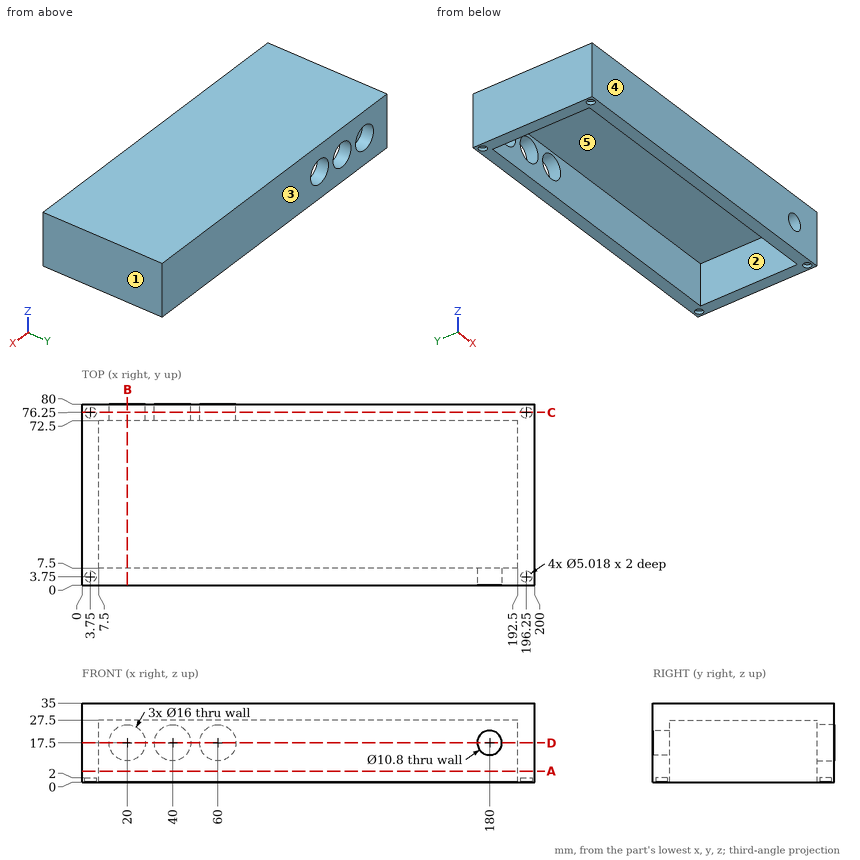
Can you work these out from the drawing? Everything is in mm from the part's minimum corner. A direction names the side the tool comes from. Give positions to 0.01 mm unless a question says otherwise; leave off trailing zeros. Loops run counter-clockwise (first coordinate to the right, second up) from the corner with the lowest first, then second, coordinate; pieces in that order, holes last. Notation, with made-up numbers: (-15, 58.5) -> (-4, 58.5) arc R11 cw to (-4, 70.5) -> close; hole circle Ø1 at (-17.5, 67). An arc over 180 degrees is marked (long way). Put each result on its own line as item: value.
(1) Please list where these lines run through material, in increasing order: probe 1 along X at (y, z) = (75.25, 17.5); probe 2 along X at (y, z) = (76.25, 0.9); probe 3 along X at (y, z) = (29, 16.5). Write a range as [from, to].
Computed:
probe 1: [0, 12], [28, 32], [48, 52], [68, 200]
probe 2: [0, 1.24], [6.26, 193.74], [198.76, 200]
probe 3: [0, 7.5], [192.5, 200]
(2) Imagine slicing it at D-D on z = 17.5. Write out the boundary of the cut face in (x, y).
Computed:
outline: (0, 0) -> (174.6, 0) -> (174.6, 7.5) -> (7.5, 7.5) -> (7.5, 72.5) -> (12, 72.5) -> (12, 80) -> (0, 80) -> close; (28, 72.5) -> (32, 72.5) -> (32, 80) -> (28, 80) -> close; (48, 72.5) -> (52, 72.5) -> (52, 80) -> (48, 80) -> close; (68, 72.5) -> (192.5, 72.5) -> (192.5, 7.5) -> (185.4, 7.5) -> (185.4, 0) -> (200, 0) -> (200, 80) -> (68, 80) -> close
(3) Imagine slicing it at C-C on y = 76.25. Write out the boundary of the cut face in (x, z), plus the area to 3 significant figures.
Computed:
outline: (0, 0) -> (1.24, 0) -> (1.24, 2) -> (6.26, 2) -> (6.26, 0) -> (193.74, 0) -> (193.74, 2) -> (198.76, 2) -> (198.76, 0) -> (200, 0) -> (200, 35) -> (0, 35) -> close; hole circle Ø16 at (20, 17.5); hole circle Ø16 at (40, 17.5); hole circle Ø16 at (60, 17.5)
area: 6,380 mm^2
(4) Imagine slicing it at A-A on z = 5. Write out the boundary of the cut face in (x, y).
Computed:
outline: (0, 0) -> (200, 0) -> (200, 80) -> (0, 80) -> close; hole (7.5, 7.5) -> (192.5, 7.5) -> (192.5, 72.5) -> (7.5, 72.5) -> close
(5) Imagine slicing it at B-B on x = 20. Write out the boundary of the cut face in (y, z).
Computed:
outline: (0, 0) -> (7.5, 0) -> (7.5, 27.5) -> (72.5, 27.5) -> (72.5, 25.5) -> (80, 25.5) -> (80, 35) -> (0, 35) -> close; (72.5, 0) -> (80, 0) -> (80, 9.5) -> (72.5, 9.5) -> close
(6) I'm going to push flat-ended pins straight in: pin 1 Ø12 at (x, z) = (137.5, 31) entering from -Y; pin 2 Ø1.5 at (x, y) = (47.5, 69) entering from -Z; pin 3 Ø1.5 at (x, y) = (195, 76) entering from -Z. Where does each tip first touch, or does it pass through?
Computed:
pin 1: y = 0
pin 2: z = 27.5
pin 3: z = 2
(7) For the marked faces 4 and 5, which set-ups out of +Z, -Z, +X, -X, +Y, -Y let a thin tool reach every point of the face, with its end or its side?
Computed:
face 4: +Z, -Z, +X, -X, -Y
face 5: -Z
(8) Thinking about a two-plate mould opening in Y: for the marked faces 1, 2 and 3, which applies, pulls with the +Y half, pulls with the -Y half, needs draft (parallel to the pull), parting line crosses it, or undercut?
Computed:
face 1: needs draft
face 2: undercut
face 3: pulls with the +Y half
